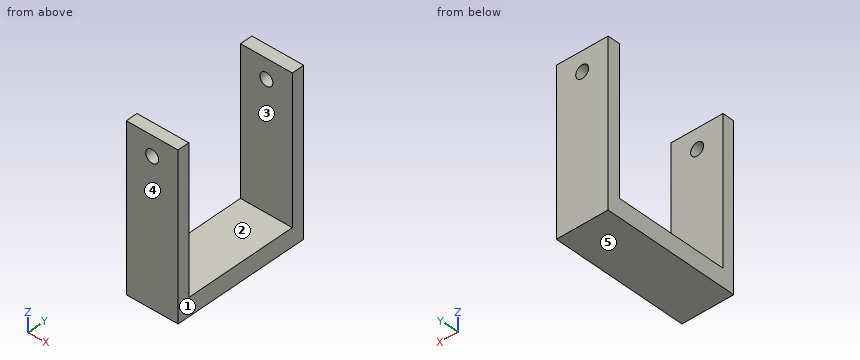
```python
from build123d import *

# Parameters (mm, degrees)
SKETCH1_W           = 20
SKETCH1_H           = 100
BOSS_EXTRUDE1_DEPTH = 53
SKETCH2_W           = 20
SKETCH2_H           = 22.115254232
CUT_EXTRUDE1_DEPTH  = 93
SKETCH3_R           = 2.5
CUT_EXTRUDE2_DEPTH  = 93
SKETCH4_W           = 20
SKETCH4_H           = 7.428579278
CUT_EXTRUDE3_DEPTH  = 93
SKETCH5_W           = 20
SKETCH5_H           = 14.111734172
CUT_EXTRUDE4_DEPTH  = 93
SKETCH6_R           = 2.5
CUT_EXTRUDE5_DEPTH  = 70
SKETCH7_W           = 20
SKETCH7_H           = 53
CUT_EXTRUDE6_DEPTH  = 37


with BuildPart() as part:
    # Sketch1 → Boss-Extrude1 (new body)
    with BuildSketch(Plane(origin=(0, 0, 0), x_dir=(1, 0, 0), z_dir=(0, 1, 0))):
        Rectangle(SKETCH1_W, SKETCH1_H)
    extrude(amount=BOSS_EXTRUDE1_DEPTH)

    # Sketch2 → Cut-Extrude1 (cut)
    with BuildSketch(Plane.XY.offset(50)):
        with Locations((0, 15.581680587)):
            Rectangle(SKETCH2_W, SKETCH2_H)
    extrude(amount=-CUT_EXTRUDE1_DEPTH, mode=Mode.SUBTRACT)

    # Sketch3 → Cut-Extrude2 (cut)
    with BuildSketch(Plane(origin=(0, 53, 0), x_dir=(1, 0, 0), z_dir=(0, 1, 0))):
        with Locations(Location((0, -43.339691346, 0), (0, 0, 270))):
            Circle(SKETCH3_R)
    extrude(amount=-CUT_EXTRUDE2_DEPTH, mode=Mode.SUBTRACT)

    # Sketch4 → Cut-Extrude3 (cut)
    with BuildSketch(Plane.XY.offset(50)):
        with Locations((0, 30.353597342)):
            Rectangle(SKETCH4_W, SKETCH4_H)
    extrude(amount=-CUT_EXTRUDE3_DEPTH, mode=Mode.SUBTRACT)

    # Sketch5 → Cut-Extrude4 (cut)
    with BuildSketch(Plane.XY.offset(50)):
        with Locations((0, 41.123754067)):
            Rectangle(SKETCH5_W, SKETCH5_H)
    extrude(amount=-CUT_EXTRUDE4_DEPTH, mode=Mode.SUBTRACT)

    # Sketch6 → Cut-Extrude5 (cut)
    with BuildSketch(Plane(origin=(0, 53, 0), x_dir=(1, 0, 0), z_dir=(0, 1, 0))):
        with Locations(Location((0, -5.385612406, 0), (0, 0, 270))):
            Circle(SKETCH6_R)
    extrude(amount=-CUT_EXTRUDE5_DEPTH, mode=Mode.SUBTRACT)

    # Sketch7 → Cut-Extrude6 (cut)
    with BuildSketch(Plane.XY.offset(50)):
        with Locations((0, 26.5)):
            Rectangle(SKETCH7_W, SKETCH7_H)
    extrude(amount=-CUT_EXTRUDE6_DEPTH, mode=Mode.SUBTRACT)


solid = part.part
```
Source: CAD feature listing. Evaluate the final solid. Frame: model axes, mm. Face numbers are marked on the shaded views. A direction names the side the tool comes from. Round coordinates to 2 decimals unless told otherwise and drop trailing zeros. Order: outer loops, then holes, each group sorted by start corner. A loop starts at its lowest first (then second) coordinate and runs counter-clockwise, first axis right, second up. Notation, with made-up numbers: (38.25, 58.5) -> (74.25, 58.5) arc R21 ccw to (74.25, 65.5) -> close; hole circle Ø1 at (44, 3.25). An arc over 180 degrees is marked (long way). One line per item, written item: value. Start each with the question number.
Q1. Section query B-B (x = -1). Return the cut outline in (y, z).
Q2. Access query for the marked faces 1 and 2. Directions: +Z, -Z, +X, -X, +Y, -Y. A direction counts if a zero-diameter tool reaches every point of the face in a straight line with its end or side. Return the directions, or none.
Q3. Section query D-D (y = 37.5). Return the cut outline in (x, z), plus the area to 3 significant figures.
Q4. Section query A-A (z = -32). Return the cut outline in (x, y), plus the area to 3 significant figures.
Q5. Draft query along Y for the marked faces 3, 4 and 5. Return one class per face: pulls with the +Y half, pulls with the -Y half, needs draft (parallel to the pull), parting line crosses it, or undercut.
Q6. Pin query (flat end, axial travel): pin 1 (10 mm diameter, centred on x = -1.5, y = 26, fed in from +Z); pin 2 (5 mm diameter, centred on y = 46, z = -17.5, fed in from -X). Return the tip coordinate at first contact, or that it passes through.
Q7. Section query C-C (x = -8). Return the cut outline in (y, z).
Q8. Material intervals for probe 1 along Y at (x, z) = (-5, 1); probe 2 along Z at (x, y) = (2, 37); probe 3 along Z at (x, y) = (-0.75, 49), sorted ascending.
Findings below:
1. outline: (0, -50) -> (53, -50) -> (53, 3.09) -> (48.18, 3.09) -> (48.18, -43) -> (4.52, -43) -> (4.52, 3.09) -> (0, 3.09) -> close; (0, 7.68) -> (4.52, 7.68) -> (4.52, 13) -> (0, 13) -> close; (48.18, 7.68) -> (53, 7.68) -> (53, 13) -> (48.18, 13) -> close
2. face 1: +Z, -Z, +X, +Y, -Y
2. face 2: +Z, +X, -X
3. outline: (-10, -50) -> (10, -50) -> (10, -43) -> (-10, -43) -> close
3. area: 140 mm²
4. outline: (-10, 0) -> (10, 0) -> (10, 4.52) -> (-10, 4.52) -> close; (-10, 48.18) -> (10, 48.18) -> (10, 53) -> (-10, 53) -> close
4. area: 187 mm²
5. face 3: undercut
5. face 4: pulls with the -Y half
5. face 5: needs draft
6. pin 1: z = -43
6. pin 2: x = -10
7. outline: (0, -50) -> (53, -50) -> (53, 13) -> (48.18, 13) -> (48.18, -43) -> (4.52, -43) -> (4.52, 13) -> (0, 13) -> close
8. probe 1: 0 to 4.52, 48.18 to 53
8. probe 2: -50 to -43
8. probe 3: -50 to 3, 7.77 to 13
